The model under review builds one solid part; all positions refer to its coordinate system, in mm. Round coordinates to 2 decimals unless told otherwise and drop trailing zeros. Write each loop counter-clockwise with the first axis right and the second up, starting at its lowest first coordinate (ties: lowest second). Pieces come first, ordered by that corner, then holes. Notation, with made-up numbers: (-36.75, 45) -> (18.25, 45) arc R27 cw to (18.25, 63) -> close; hole circle Ø7 at (56.5, 34). An arc over 180 degrees is marked (long way). Use CSV: the item, a comma, the result in double quotes. Start each with the question number.
1) For pin 1 Ø6 at (x, y) = (64.5, 29) entering from -Z; pin 2 Ø0.9 at (x, z) = (141.5, 1) entering from +Y; pin 3 Ø0.9 at (x, z) = (315.5, 1) entering from +Y; pin 4 Ø1.5 at (x, z) = (100.5, 1.5) entering from -Y, all flat-tipped, find the tip position at first contact; note any pin that passes through.
2) Wall thickness on probe 1 along Y at (x, z) = (115.5, 0.3); probe 2 along Y at (x, z) = (16.5, 1.6); probe 3 along Y at (x, z) = (330, 0.95): over which ranges is each line inside the solid? List them lowest first. Write a range as [from, to].
3) Take a section at B-B, the plane x = 205.5. Give the boundary of the cut face in (y, z), then the cut area to 3 significant figures.
4) Take a section at C-C, the plane x = 241. Give the boundary of the cut face in (y, z).
5) Take a section at A-A, the plane z = 1.2. State how many separate pieces and enclosed holes the cut face has, then the cut area to 3 significant figures.
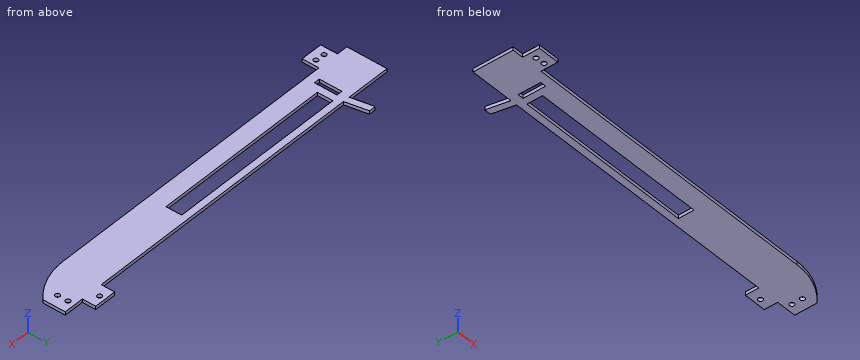
Autodesk Inventor part; units mm, degrees
ref_plane "YZ Plane" through (0, 0, 0) normal (1, 0, 0) x (0, 1, 0)
ref_plane "XZ Plane" through (0, 0, 0) normal (0, 1, 0) x (-1, 0, 0)
ref_plane "XY Plane" through (0, 0, 0) normal (0, 0, 1) x (1, 0, 0)
sketch "Sketch1" plane through (0, 0, 0) normal (0, 0, 1) x (1, 0, 0)
  line L0 (0, 0) -> (300, 0)
  line L1 (300, 0) -> (300, 16)
  line L2 (300, 16) -> (0, 16)
  line L3 (0, 16) -> (0, 0)
  line L4 (0, 0) -> (22.0483, 0)
  line L5 (10, 0) -> (29.5, 0)
  line L6 (29.5, 0) -> (29.5, -15)
  line L7 (29.5, -15) -> (10, -15)
  line L8 (10, -15) -> (10, 0)
  point P0 (0, 8)
  dimension "d2" = 19.5
  dimension "d3" = 15
  dimension "d4" = 10
  dimension "d5" = 16
  dimension "d8" = 300
extrude "Extrusion1" add sketch "Sketch1" along normal blind 3
sketch "Sketch2" plane through (0, 0, 3) normal (0, 0, 1) x (1, 0, 0)
  line L0 (0, 16) -> (0, 0)
  line L1 (0, 16) -> (0, 36)
  line L2 (300, 0) -> (300, 16)
  line L3 (340, 16) -> (340, 36)
  line L4 (340, 36) -> (0, 36)
  line L5 (300, 16) -> (0, 16)
  line L6 (50, 16) -> (50, 30)
  line L7 (50, 30) -> (210, 30)
  line L8 (210, 30) -> (210, 16)
  line L9 (40, 36) -> (36, 56)
  line L10 (36, 56) -> (42, 56)
  line L11 (42, 56) -> (46, 36)
  circle A0 centre (330, 30) radius 2.1
  circle A1 centre (330, 20.6) radius 2.1
  line L12 (340, 16) -> (300, 16)
  line L13 (302, 36) -> (322, 36)
  line L14 (322, 36) -> (322, 48)
  line L15 (322, 48) -> (302, 48)
  line L16 (302, 48) -> (302, 36)
  circle A2 centre (312, 43) radius 2.075
  point P0 (312, 48)
  point P1 (322, 36)
  dimension "d44" = 20
  dimension "d45" = 160
  dimension "d46" = 50
  dimension "d47" = 14
  dimension "d48" = 20
  dimension "d49" = 6
  dimension "d50" = 4
  dimension "d51" = 40
  dimension "d83" = 4.2
  dimension "d84" = 4.2
  dimension "d85" = 6
  dimension "d86" = 9.4
  dimension "d87" = 10
  dimension "d99" = 40
  dimension "d107" = 7
  dimension "d108" = 20
  dimension "d109" = 12
  dimension "d110" = 18
  dimension "d111" = 4.15
extrude "Extrusion2" add sketch "Sketch2" against normal blind 3 contours L1 L4 L3 L12 L5 L8 L7 L6 | L9 L10 L11 L4 | L16 L15 L14 L4
sketch "Sketch3" plane through (0, 0, 3) normal (0, 0, 1) x (1, 0, 0)
  circle A0 centre (16.5, -6.5) radius 2.1
  circle A1 centre (24.5, -7) radius 2.1
  line L0 (29.5, 0) -> (300, 0)
  line L1 (29.5, -15) -> (29.5, 0)
  point P0 (0, 0)
  dimension "d75" = 4.2
  dimension "d76" = 6.5
  dimension "d77" = 4.2
  dimension "d78" = 7
  dimension "d79" = 5
  dimension "d80" = 8
extrude "Extrusion3" cut sketch "Sketch3" against normal blind 3
sketch "Sketch4" plane through (0, 0, 3) normal (0, 0, 1) x (1, 0, 0)
  line L0 (29.5, 0) -> (300, 0)
  circle A0 centre (41, 18) radius 2.6
  line L1 (340, 36) -> (46, 36)
  line L2 (38.4, 28.1) -> (43.6, 28.1)
  line L3 (43.6, 28.1) -> (43.6, 7.9)
  line L4 (43.6, 7.9) -> (38.4, 7.9)
  line L5 (38.4, 7.9) -> (38.4, 28.1)
  line L6 (38.4, 28.1) -> (43.6, 7.9) construction
  line L7 (43.6, 28.1) -> (38.4, 7.9) construction
  point P0 (0, 0)
  point P1 (43.6, 18)
  point P2 (38.4, 18)
  dimension "d95" = 18
  dimension "d96" = 5.2
  dimension "d100" = 5
  dimension "d101" = 20.2
extrude "Extrusion4" cut sketch "Sketch4" against normal blind 3
sketch "Sketch5" plane through (0, 0, 3) normal (0, 0, 1) x (1, 0, 0)
  line L0 (29.5, 0) -> (300, 0)
  line L1 (340, 36) -> (340, 16)
  arc A0 (300, 0) -> (340, 16) centre (300, 58) ccw
  line L2 (300, 0) -> (300, 16)
  line L3 (300, 0) -> (300, 16)
  line L4 (300, 16) -> (340, 16)
  point P0 (0, 0)
extrude "Extrusion5" add sketch "Sketch5" against normal blind 3
properties part number "Middle_bar"
Values found:
1,pin 1,"z = 0"
1,pin 2,"y = 36"
1,pin 3,"y = 48"
1,pin 4,"y = 0"
2,probe 1,"[0, 16], [30, 36]"
2,probe 2,"[-15, -8.6], [-4.4, 36]"
2,probe 3,"[8.36, 18.5], [22.7, 27.9], [32.1, 36]"
3,outline,"(0, 0) -> (16, 0) -> (16, 3) -> (0, 3) -> close; (30, 0) -> (36, 0) -> (36, 3) -> (30, 3) -> close"
3,area,"66.0 mm²"
4,outline,"(0, 0) -> (36, 0) -> (36, 3) -> (0, 3) -> close"
5,separate pieces,"1"
5,enclosed holes,"7"
5,area,"10,300 mm²"
